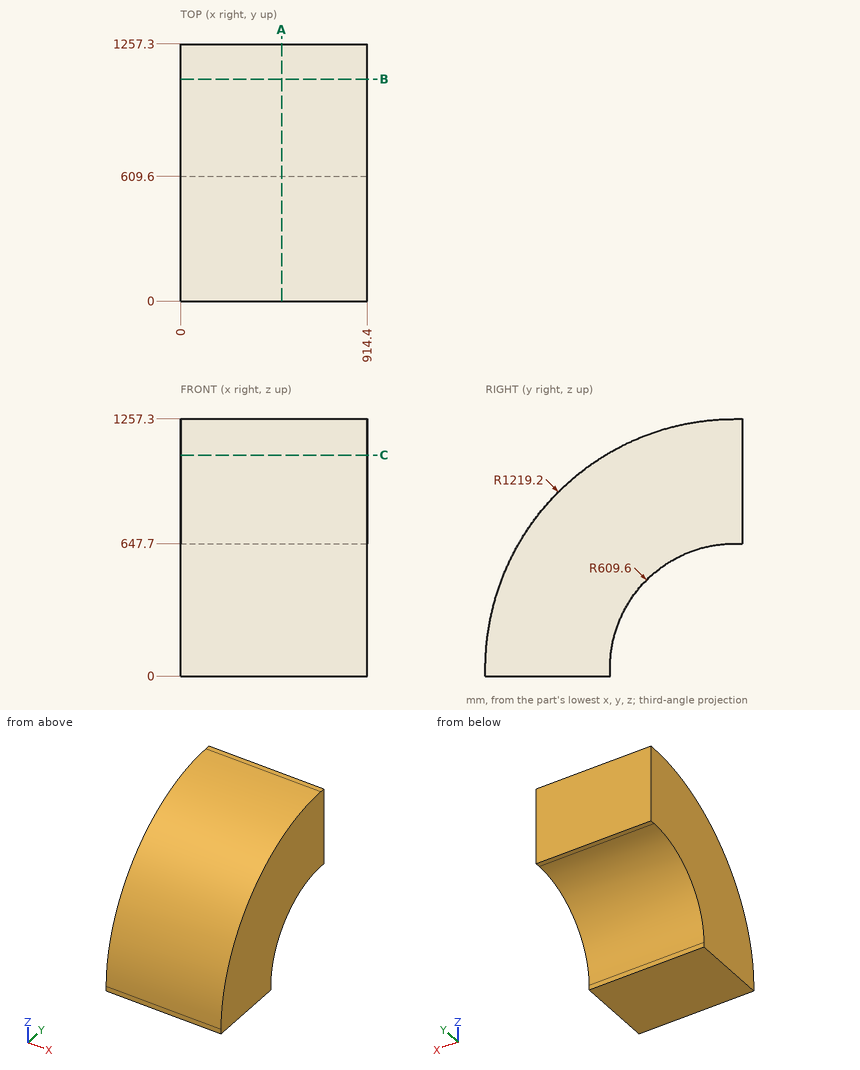
Part print with two shaded views. Sizes in mm from the minimum x, y, z corner. Coordinates: 2 decimals unless noted, no trailing zeros. Write each loop counter-clockwise with the first axis right and the second up, starting at its lowest first coordinate (ties: lowest second). Pieces come first, ordered by that corner, then holes. Notation, with made-up numbers: (-33, 2) - (16, 2) arc R10 cw to (16, 15) - close; hole circle Ø3 at (77.25, 72). An arc over 180 degrees is marked (long way). Use a Markdown table: item, result. Add a question column.
Item 1: Band-saw the part on C-C, the plane z = 1081. Write the cut outline in (x, y), and give its area (3 significant figures).
Item 2: Drill centre lines: line 1 along Y through (x, z) = (642.5, 57); line 2 along Y through (x, z) = (494.5, 987); line 3 along Z through (x, y) = (487, 950). Where is each one in solid material? Low to high.
Item 3: Band-saw the part on A-A, the plane x = 495. Write the cut outline in (y, z).
Item 4: Drop flat-ended pins along their axis: pin 1 (10 mm diameter, centred on x = 111.5, y = 195.5, fed in from -Z); pin 2 (19 mm diameter, centred on x = 251, z = 27.5, fed in from +Y); pin 3 (4 mm diameter, centred on x = 694.5, y = 497, fed in from +Z); pin 4 (1.5 mm diameter, centred on x = 506, y = 1061, fed in from -Z). Give the stop position or say it passes through.
Item 5: Band-saw the part on B-B, the plane y = 1086. Write the cut outline in (x, z).
A:
| question | item | result |
|---|---|---|
| 1 | outline | (0, 587.69) - (914.4, 587.69) - (914.4, 1257.3) - (0, 1257.3) - close |
| 1 | area | 612,000 mm² |
| 2 | line 1 | y = 0.15 to 609.89 |
| 2 | line 2 | y = 453.67 to 1257.3 |
| 2 | line 3 | z = 585.04 to 1227.21 |
| 3 | outline | (0, 0) - (609.6, 0) - (609.6, 38.1) arc R609.6 cw to (1219.2, 647.7) - (1257.3, 647.7) - (1257.3, 1257.3) - (1219.2, 1257.3) arc R1219.2 ccw to (0, 38.1) - close |
| 4 | pin 1 | stops at z = 0 |
| 4 | pin 2 | stops at y = 609.6 |
| 4 | pin 3 | stops at z = 1021.85 |
| 4 | pin 4 | stops at z = 626.61 |
| 5 | outline | (0, 632.97) - (914.4, 632.97) - (914.4, 1250) - (0, 1250) - close |
